```python
from build123d import *

# Parameters (mm, degrees)
BOSS_EXTRUDE1_DEPTH = 2.5
SKETCH1_3_R         = 3.25
BOSS_EXTRUDE2_DEPTH = 17.5
SKETCH1_4_R         = 3.25
BOSS_EXTRUDE3_DEPTH = 17.5


with BuildPart() as part:
    # Sketch1 → Boss-Extrude1 (new, symmetric)
    with BuildSketch(Plane.XY):
        with BuildLine():
            Line((7.5, 0), (7.5, -53))
            ThreePointArc((7.5, -53), (0, -60.5), (-7.5, -53))
            Line((-7.5, -53), (-7.5, 0))
            ThreePointArc((-7.5, 0), (0, 7.5), (7.5, 0))
        make_face()
    extrude(amount=BOSS_EXTRUDE1_DEPTH, both=True)

    # Sketch1_3 → Boss-Extrude2 (add)
    with BuildSketch(Plane.XY):
        Circle(SKETCH1_3_R)
    extrude(amount=-BOSS_EXTRUDE2_DEPTH)

    # Sketch1_4 → Boss-Extrude3 (add)
    with BuildSketch(Plane.XY):
        with Locations((0, -53)):
            Circle(SKETCH1_4_R)
    extrude(amount=BOSS_EXTRUDE3_DEPTH)


solid = part.part
```
Geometry: final body of the model. Coordinates: model frame, mm. A direction names the side the tool comes from. Round coordinates to 2 decimals unless told otherwise and drop trailing zeros. Write each loop counter-clockwise with the first axis right and the second up, starting at its lowest first coordinate (ties: lowest second). Pieces come first, ordered by that corner, then holes.
Item 1: Section query A-A (x = 0). Return loops of the section in (y, z), plus the area to 3 significant figures.
Item 2: Material intervals for L1, parallel to Z at x = -5.75, y = -35.5; L2, parallel to Z at x = -0.5, y = -1; L3, parallel to Y at x = -1.75, z = 16.5, sorted ascending.
Item 3: Section query B-B (y = -20.5). Return loops of the section in (x, z), plus the area to 3 significant figures.
Item 4: Set-up query: faces 1 (the face through (-2.579, -1.978, -9.895)), 2 (the face through (-0.705, -56.173, 9.895)), 3 (the face through (0.16, -60.5, 0.04)). Return all of +Z, -Z, +X, -X, +Y, -Y with unobstructed straight access to the full face (end or side cutting, diameter ignored); none if empty.
Item 5: Section query C-C (z = 11). Return loops of the section in (x, y).
Item 6: Pin query (flat end, axial travel): P1, Ø3, axis at y = -7.5, z = 4.5, coming from the -X side; P2, Ø3, axis at x = 1, y = -38, coming from the -Z side; P3, Ø2, axis at x = -1.5, z = 6.5, coming from the +Y side; P4, Ø2, axis at x = -2.5, z = 5, coming from the +Y side. Return the tip coordinate at first contact, or that it passes through.
Item 7: Section query D-D (x = 4.5). Return loops of the section in (y, z).
Completed:
1. outline: (-60.5, -2.5) - (-3.25, -2.5) - (-3.25, -17.5) - (3.25, -17.5) - (3.25, -2.5) - (7.5, -2.5) - (7.5, 2.5) - (-49.75, 2.5) - (-49.75, 17.5) - (-56.25, 17.5) - (-56.25, 2.5) - (-60.5, 2.5) - close
1. area: 535 mm2
2. L1: z = -2.5 to 2.5
2. L2: z = -17.5 to 2.5
2. L3: y = -55.74 to -50.26
3. outline: (-7.5, -2.5) - (7.5, -2.5) - (7.5, 2.5) - (-7.5, 2.5) - close
3. area: 75.0 mm2
4. face 1: -Z
4. face 2: +Z
4. face 3: +Z, -Z, -Y
5. outline: circle Ø6.5 at (0, -53)
6. P1: passes through
6. P2: stops at z = -2.5
6. P3: stops at y = -49.79
6. P4: stops at y = -50.12
7. outline: (-59, -2.5) - (6, -2.5) - (6, 2.5) - (-59, 2.5) - close
